Model file for the job. Use its own axes, mm. A direction names the side the tool comes from. Round coordinates to 2 decimals unless told otherwise and drop trailing zeros. Loops run counter-clockwise (first coordinate to the right, second up) from the corner with the lowest first, then second, coordinate; pieces in that order, holes last. Notation, with made-up numbers: M -24,63 L -5,63 A33 ccw -5,99 Z; hole C 17.5,0 d9. An arc over 180 degrees is marked long. Use a Markdown table: item, result. Add a question column.
Item 1: Saw through at B-B on z = 25. Write the cut outline in (x, y), then the cut area to 3 significant figures.
Item 2: Saw through at A-A on y = 0. Write the cut outline in (x, z).
Item 3: Two-plate mould, pull along Y, no slides. Class faces 1 (the flat face through (99, -25, 19)), 2 (the flat face through (151, 31, 50)), 3 (the flat face through (12, 87.5, -6)): +Y half, -Y half, draft (parallel to the pull), parting line (faces both ways), or undercut.
Item 4: Saw through at D-D on z = 47. Write the cut outline in (x, y), then the cut area to 3 significant figures.
Item 5: Wall check: L1, parallel to Y at x = 162, z = 23; L2, parallel to Y at x = 150, z = 56; L3, parallel to X at y = 33.5, z = 47. Give the ranges that are in metal, low to high. Write a range as from..to.
Item 6: Saw through at C-C on x = 150. Write the cut outline in (y, z).
Item 7: Tool access for faces 4 (the flat face through (0, 40, 5)), 5 (the flat face through (149, 15.5, 44)), 6 (the flat face through (12, -31, -12)), 7 (the flat face through (74, -63, 6)), 8 (the flat face through (25, -59, -12)): list every direction of +Z, -Z, +X, -X, +Y, -Y with a clear straight run to the whole face (end or side of a thin tool).
Item 8: Pin check, flat tips, straight feed: P1, Ø11.5, axis at x = 67, z = 23.5, coming from the +Y side; P2, Ø3, axis at x = 155, z = 45.5, coming from the -Y side; P3, Ø10, axis at x = 95, y = -58, coming from the -Z side. Stop position of each tip, or through.
```python
from build123d import *

# Parameters (mm, degrees)
PAD_DEPTH       = 62
SKETCH001_W     = 174.899156
SKETCH001_H     = 58.891647
SKETCH001_W_2   = 149.195125
SKETCH001_H_2   = 63.358872
POCKET_DEPTH    = 50
SKETCH002_W     = 24.450794
SKETCH002_H     = 18.2717568888
SKETCH002_W_2   = 25.01263
POCKET001_DEPTH = 200.001
SKETCH003_W     = 109.462605
SKETCH003_H     = 100.191001
POCKET002_DEPTH = 12
SKETCH004_W     = 50
SKETCH004_H     = 111.170834
POCKET003_DEPTH = 12
SKETCH005_W     = 25
SKETCH005_H     = 175
PAD001_DEPTH    = 25
POCKET004_DEPTH = 200.001
SKETCH007_W     = 31
SKETCH007_H     = 12
POCKET005_DEPTH = 100.001
SKETCH008_R     = 12.5
POCKET006_DEPTH = 87.001
SKETCH009_W     = 25.552227
SKETCH009_H     = 12
POCKET007_DEPTH = 75.001


with BuildPart() as part:
    # Sketch → Pad (new body)
    with BuildSketch(Plane.XY):
        Polygon((0, 87.5), (0, -87.5), (25, -87.5), (125, -37.5), (200, -37.5), (200, 37.5), (125, 37.5), (25, 87.5), align=None)
    extrude(amount=PAD_DEPTH)

    # Sketch001 → Pocket (cut)
    with BuildSketch(Plane.XY.offset(62)):
        with Locations((66.856742, 66.9458235)):
            Rectangle(SKETCH001_W, SKETCH001_H)
        with Locations((63.5040375, -69.179436)):
            Rectangle(SKETCH001_W_2, SKETCH001_H_2)
    extrude(amount=-POCKET_DEPTH, mode=Mode.SUBTRACT)

    # Sketch002 → Pocket001 (cut, through all)
    with BuildSketch(Plane.YZ.offset(200)):
        with Locations((-37.225397, 59.1358784444)):
            Rectangle(SKETCH002_W, SKETCH002_H)
        with Locations((37.506315, 59.1358784444)):
            Rectangle(SKETCH002_W_2, SKETCH002_H)
    extrude(amount=-POCKET001_DEPTH, mode=Mode.SUBTRACT)

    # Sketch003 → Pocket002 (cut)
    with BuildSketch(Plane.XY.offset(62)):
        with Locations((45.2686975, 1.1479225)):
            Rectangle(SKETCH003_W, SKETCH003_H)
    extrude(amount=-POCKET002_DEPTH, mode=Mode.SUBTRACT)

    # Sketch004 → Pocket003 (cut)
    with BuildSketch(Plane.XY.offset(50)):
        with Locations((75, 0.690428)):
            Rectangle(SKETCH004_W, SKETCH004_H)
    extrude(amount=-POCKET003_DEPTH, mode=Mode.SUBTRACT)

    # Sketch005 → Pad001 (new body)
    with BuildSketch(Plane(origin=(0, 0, 0), x_dir=(1, 0, 0), z_dir=(0, 0, -1))):
        with Locations((12.5, 0)):
            Rectangle(SKETCH005_W, SKETCH005_H)
    extrude(amount=PAD001_DEPTH)

    # Sketch006 → Pocket004 (cut, through all)
    with BuildSketch(Plane(origin=(0, 0, 0), x_dir=(0, -1, 0), z_dir=(-1, 0, 0))):
        Polygon((-25, 38), (25, 38), (25, 0), (31, 0), (31, -41.126076), (-31, -41.126076), (-31, 0), (-25, 0), align=None)
    extrude(amount=-POCKET004_DEPTH, mode=Mode.SUBTRACT)

    # Sketch007 → Pocket005 (cut, through all)
    with BuildSketch(Plane(origin=(100, 0, 0), x_dir=(0, -1, 0), z_dir=(-1, 0, 0))):
        with Locations((0, 44)):
            Rectangle(SKETCH007_W, SKETCH007_H)
    extrude(amount=-POCKET005_DEPTH, mode=Mode.SUBTRACT)

    # Sketch008 → Pocket006 (cut, through all)
    with BuildSketch(Plane.XY.offset(62)):
        with Locations((150, 0)):
            Circle(SKETCH008_R)
    extrude(amount=-POCKET006_DEPTH, mode=Mode.SUBTRACT)

    # Sketch009 → Pocket007 (cut, through all)
    with BuildSketch(Plane.XY.offset(50)):
        with Locations((50.7761135, 0)):
            Rectangle(SKETCH009_W, SKETCH009_H)
    extrude(amount=-POCKET007_DEPTH, mode=Mode.SUBTRACT)


solid = part.part
```
Entries:
| question | item | result |
|---|---|---|
| 1 | outline | M 0,-37.5 L 200,-37.5 L 200,-25 L 0,-25 Z; M 0,25 L 200,25 L 200,37.5 L 0,37.5 Z |
| 1 | area | 5,000 mm2 |
| 2 | outline | M 0,38 L 38,38 L 38,50 L 0,50 Z; M 100,50 L 137.5,50 L 137.5,62 L 100,62 Z; M 162.5,50 L 200,50 L 200,62 L 162.5,62 Z |
| 3 | face 1 | undercut |
| 3 | face 2 | draft |
| 3 | face 3 | +Y half |
| 4 | outline | M 0,-37.5 L 50,-37.5 L 50,-6 L 38,-6 L 38,6 L 50,6 L 50,37.5 L 0,37.5 Z; M 100,-37.5 L 200,-37.5 L 200,-15.5 L 100,-15.5 Z; M 100,15.5 L 200,15.5 L 200,37.5 L 100,37.5 Z |
| 4 | area | 8,010 mm2 |
| 5 | L1 | -37.5..-25, 25..37.5 |
| 5 | L2 | -25..-12.5, 12.5..25 |
| 5 | L3 | 0..50, 100..200 |
| 6 | outline | M -37.5,0 L -25,0 L -25,38 L -15.5,38 L -15.5,50 L -12.5,50 L -12.5,62 L -25,62 L -25,50 L -37.5,50 Z; M 12.5,50 L 15.5,50 L 15.5,38 L 25,38 L 25,0 L 37.5,0 L 37.5,50 L 25,50 L 25,62 L 12.5,62 Z |
| 7 | face 4 | +Z, -Z, -X, +Y, -Y |
| 7 | face 5 | -Z, +X |
| 7 | face 6 | -Z, +X, -X |
| 7 | face 7 | +Z, -Z, +X, -Y |
| 7 | face 8 | -Z, +X, +Y, -Y |
| 8 | P1 | y = 37.5 |
| 8 | P2 | y = -37.5 |
| 8 | P3 | z = 0 |
